Could you check a few things on this drawing? It's one solid part, dimensions in mm from its lowest x, y, z. Give positions to 0.01 mm unless a question says otherwise; leave off trailing zeros. Order: outer loops, then holes, each group sorted by start corner. A loop starts at its lowest first (then second) coordinate and runs counter-clockwise, first axis right, second up.
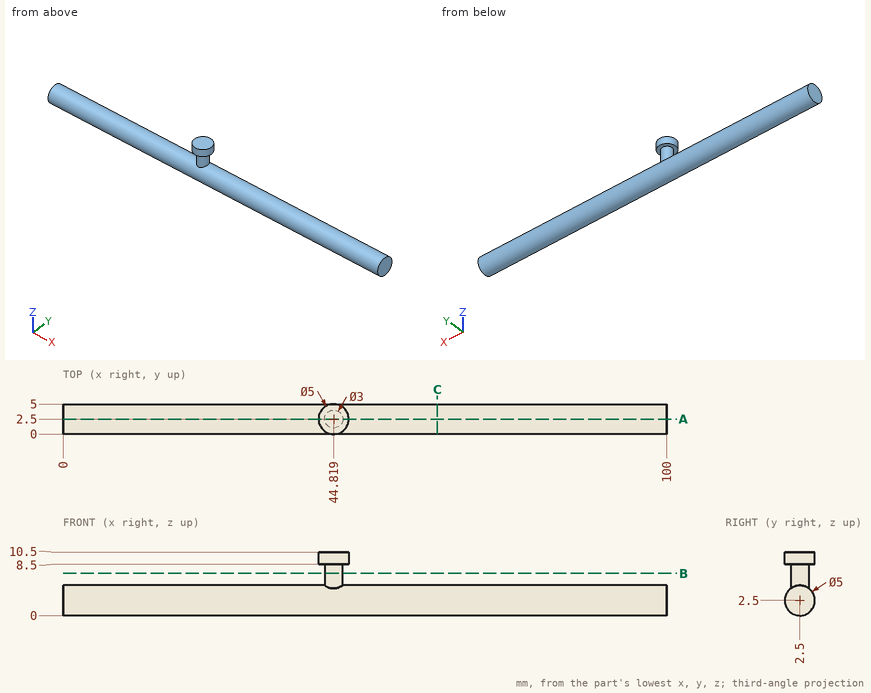
1) If I drill on line 1 (Y direction, x = 45, z = 2.75); line 2 (Z direction, x = 70, y = 2.5); line 3 (Z direction, x = 56.5, y = 3.65), over which ranges is the centre line in solid material (lowest first)?
2) I'm going to push flat-ended pins straight in: pin 1 Ø4 at (x, z) = (79, 5) entering from -Y; pin 2 Ø2 at (x, z) = (35, 1) entering from +Y; pin 3 Ø1.5 at (x, y) = (88.5, 1) entering from -Z (1 decimal). Where does each tip first touch, or does it pass through?
3) Suppose I cut it at A-A (y = 2.5). Please give me the cut outline in (x, z).
4) Suppose I cut it at C-C (x = 62). Please give me the cut outline in (y, z), and give its area (3 significant figures).
5) Suppose I cut it at B-B (z = 7). Please give me the cut outline in (x, y).
Results:
1. line 1: y = 0.01 to 4.99
1. line 2: z = 0 to 5
1. line 3: z = 0.28 to 4.72
2. pin 1: stops at y = 0.05
2. pin 2: stops at y = 4.95
2. pin 3: stops at z = 0.1
3. outline: (0, 0) - (100, 0) - (100, 5) - (46.32, 5) - (46.32, 8.5) - (47.32, 8.5) - (47.32, 10.5) - (42.32, 10.5) - (42.32, 8.5) - (43.32, 8.5) - (43.32, 5) - (0, 5) - close
4. outline: circle Ø5 at (2.5, 2.5)
4. area: 19.6 mm2
5. outline: circle Ø3 at (44.82, 2.5)
